Build history of the part. All positions in model axes, mm. A direction names the side the tool comes from. Give positions to 0.01 mm unless a question says otherwise; leave off trailing zeros. Order: outer loops, then holes, each group sorted by start corner. A loop starts at its lowest first (then second) coordinate and runs counter-clockwise, first axis right, second up. Notation, with made-up numbers: (7, 57) - (61, 57) arc R21 cw to (61, 85) - close; hole circle Ø2 at (16, 60.5). An arc over 180 degrees is marked (long way). Write each question's results on one line, items separated by ' | '. Start each with the question number.
1) Cut at A-A on z = 0. List the corners of the cut face in (x, y) (3 decimals).
2) Cut at C-C on x = -27.75. List the corners of the cut face in (y, z).
3) Two-plate mould, pull along X, no slides. Class faces 1 (the face through (-30, 0, 0)), 2 (the face through (-28.937, 3.027, -3.948)), 3 (the face through (-27.56, -4.05, 2.58)): +X half, -X half, draft (parallel to the pull), parting line (faces both ways), or undercut.
4) Drill centre lines: line 1 along Y through (x, z) = (-19, -0.5); line 2 along X through (y, z) = (5, 5). Where is each one in solid material? Low to high. Write a range as from..to.
5) Cut at D-D on x = -22. List the corners of the cut face in (y, z), plus the area to 3 significant figures.
6) Drop flat-ended pins along their axis: pin 1 Ø3 at (y, z) = (-5.5, 5) entering from -X; pin 2 Ø5 at (x, y) = (-16, 0) entering from +Z; pin 3 Ø5 at (x, y) = (-3.5, 3) entering from -Z. Give the stop position or say it passes through.
7) Tool access for faces 4 (the face through (0, 0, 0)), 5 (the face through (-14.8, 4.88, -1.08)): list every direction of +Z, -Z, +X, -X, +Y, -Y with a clear straight run to the whole face (end or side of a thin tool).
from build123d import *

# Parameters (mm, degrees)
F2_SIZE = 0.25


with BuildPart() as f1:
    # F0 (on Front) → F1 (revolve)
    with BuildSketch(Plane.XZ):
        Polygon((-30, 0), (0, 0), (0, 7.5), (-2, 7.5), (-2, 5), (-27, 5), (-27, 4.8), (-28.1, 4.8), (-28.1, 4.975), (-30, 4.975), align=None)
    revolve(axis=Axis((2.79349, 0, 0), (1, 0, 0)))

    # F2
    f2_edges = [f1.edges().sort_by_distance(p)[0] for p in [
        (-2, 0, -7.5),
        (-2, 0, -5),
        (0, 0, -7.5),
        (-30, 0, -4.975),
    ]]
    chamfer(f2_edges, length=F2_SIZE)


solid = f1.part
Results:
1) outline: (-30, -4.725) - (-29.75, -4.975) - (-28.1, -4.975) - (-28.1, -4.8) - (-27, -4.8) - (-27, -5) - (-2.25, -5) - (-2, -5.25) - (-2, -7.25) - (-1.75, -7.5) - (-0.25, -7.5) - (0, -7.25) - (0, 7.25) - (-0.25, 7.5) - (-1.75, 7.5) - (-2, 7.25) - (-2, 5.25) - (-2.25, 5) - (-27, 5) - (-27, 4.8) - (-28.1, 4.8) - (-28.1, 4.975) - (-29.75, 4.975) - (-30, 4.725) - close
2) outline: circle Ø9.6 at (0, 0)
3) face 1: -X half | face 2: draft | face 3: undercut
4) line 1: -4.97..4.97 | line 2: -2..0
5) outline: circle Ø10 at (0, 0) | area: 78.5 mm^2
6) pin 1: x = -2 | pin 2: z = 5 | pin 3: z = -7.4
7) face 4: +Z, -Z, +X, +Y, -Y | face 5: -X
